Geometry check sheet. Reference: the model listing, model coordinates, mm. Give positions to 0.01 mm unless a question says otherwise; leave off trailing zeros. Order: outer loops, then holes, each group sorted by start corner. A loop starts at its lowest first (then second) coordinate and runs counter-clockwise, first axis right, second up.
from build123d import *

# Parameters (mm, degrees)
SKETCH1_W           = 10
SKETCH1_H           = 10
BOSS_EXTRUDE1_DEPTH = 3
SKETCH2_R           = 3.175
CUT_EXTRUDE1_DEPTH  = 10
FILLET1_RADIUS      = 5
FILLET1_LENGTH      = 3
FILLET2_R           = 5


with BuildPart() as part:
    # Sketch1 → Boss-Extrude1 (new body)
    with BuildSketch(Plane(origin=(0, 0, 0), x_dir=(0, 0, -1), z_dir=(1, 0, 0))):
        Rectangle(SKETCH1_W, SKETCH1_H)
    extrude(amount=BOSS_EXTRUDE1_DEPTH)

    # Sketch2 → Cut-Extrude1 (cut)
    with BuildSketch(Plane.ZY):
        Circle(SKETCH2_R)
    extrude(amount=-CUT_EXTRUDE1_DEPTH, mode=Mode.SUBTRACT)

    # Fillet1: full round fillet: the end face becomes a half cylinder, R = half its width
    fillet1_face = Plane((1.5, 5, 0), x_dir=(1, 0, 0), z_dir=(0, 1, 0))  # on the end face: x along it, z out of the body
    fillet1_slab = fillet1_face.offset(-FILLET1_RADIUS / 2) * Box(FILLET1_LENGTH, 2 * FILLET1_RADIUS, FILLET1_RADIUS, mode=Mode.PRIVATE)  # the body's end, R deep
    fillet1_round = Plane((1.5, 0, 0), x_dir=(0, 1, 0), z_dir=(1, 0, 0)) * Cylinder(FILLET1_RADIUS, FILLET1_LENGTH, mode=Mode.PRIVATE)  # its axis R under the face
    add(fillet1_slab - fillet1_round, mode=Mode.SUBTRACT)

    # Fillet2
    fillet2_edges = [part.edges().sort_by_distance(p)[0] for p in [
        (1.5, -5, -5),
        (1.5, -5, 5),
    ]]
    fillet(fillet2_edges, radius=FILLET2_R - 0.0001)  # a hair under: the kernel refuses the full size


solid = part.part
Item 1: Sectioned sample at D-D (y = -4). Enter the section's corners in (x, z).
Reported:
outline: (0, -3) - (3, -3) - (3, 3) - (0, 3) - close
Item 2: Sectioned sample at B-B (z = -1). Enter the section's corners in (x, y), and give its area (3 significant figures).
Reported:
outline: (0, -4.9) - (3, -4.9) - (3, -3.01) - (0, -3.01) - close; (0, 3.01) - (3, 3.01) - (3, 4.9) - (0, 4.9) - close
area: 11.3 mm2
Item 3: Scan lines: L1, parallel to Y at x = 0.65, z = 0 (3 decimals); L2, parallel to Z at x = 2.85, y = 2; L3, parallel to Y at x = 1.6, z = -2.25. Record each from-to range of solid material in increasing order.
Reported:
L1: y = -5 to -3.175, 3.175 to 5
L2: z = -4.58 to -2.47, 2.47 to 4.58
L3: y = -4.47 to -2.24, 2.24 to 4.47
Item 4: Sectioned sample at C-C (y = 1.5). Enter the section's corners in (x, z).
Reported:
outline: (0, -4.77) - (3, -4.77) - (3, -2.8) - (0, -2.8) - close; (0, 2.8) - (3, 2.8) - (3, 4.77) - (0, 4.77) - close
Item 5: Gauge pin test, flat ends, axial feed: pin 1 (1 mm diameter, centred on x = 1, z = 2.5, fed in from -Y); pin 2 (1 mm diameter, centred on y = -3, z = -1, fed in from -X); pin 3 (1.5 mm diameter, centred on x = 0.5, z = 3, fed in from +Y); pin 4 (5 mm diameter, centred on y = 0, z = 0, fed in from +X). Record the tip position at first contact, or that the pin passes through.
Reported:
pin 1: stops at y = -4.58
pin 2: stops at x = 0
pin 3: stops at y = 4.47
pin 4: passes through
Item 6: Draft check along Z on faces 1 (the cylindrical face through (2, 5, 0)), 2 (the cylindrical face through (1.48, -3.1, -0.69)), 3 (the cylindrical face through (2, -4, -3)). Enter one of: released by +Z, released by -Z, zero draft, split by the parting line, or undercut.
Reported:
face 1: split by the parting line
face 2: undercut
face 3: released by -Z
